```python
from build123d import *

# Parameters (mm, degrees)
BOSS_EXTRUDE1_DEPTH = 6.5
SKETCH4_R           = 1.5875
CUT_EXTRUDE1_DEPTH  = 10
SKETCH5_R           = 1.5875
CUT_EXTRUDE2_DEPTH  = 10


with BuildPart() as part:
    # Sketch3 → Boss-Extrude1 (new body, symmetric)
    with BuildSketch(Plane.XY):
        Polygon((3.175, -3.175), (-4.7625, -3.175), (-4.7625, -4.7625), (4.7625, -4.7625), (4.7625, 4.7625), (3.175, 4.7625), align=None)
    extrude(amount=BOSS_EXTRUDE1_DEPTH, both=True)

    # Sketch4 → Cut-Extrude1 (cut)
    with BuildSketch(Plane(origin=(4.7625, 0, 0), x_dir=(0, 0, -1), z_dir=(1, 0, 0))):
        with Locations((3, 1.2375)):
            Circle(SKETCH4_R)
    extrude(amount=-CUT_EXTRUDE1_DEPTH, mode=Mode.SUBTRACT)

    # Sketch5 → Cut-Extrude2 (cut)
    with BuildSketch(Plane.XZ.offset(4.7625)):
        with Locations((-1.2375, 3)):
            Circle(SKETCH5_R)
    extrude(amount=-CUT_EXTRUDE2_DEPTH, mode=Mode.SUBTRACT)


solid = part.part
```
Work out the finished part from the listing and answer in its coordinate system (mm). A direction names the side the tool comes from. Coordinates: 2 decimals unless noted, no trailing zeros. Write each loop counter-clockwise with the first axis right and the second up, starting at its lowest first coordinate (ties: lowest second). Pieces come first, ordered by that corner, then holes.
Q1. Which of the six approach directions +Z, -Z, +X, -X, +Y, -Y give full straight-line access (tool end or side, diameter ignored) to faces 1 (the face through (3.175, 1, 0)), 2 (the face through (4, 4.762, 0))?
Q2. Each of these flat-tipped pins is pushed along its axis until it touches: pin 1 Ø4 at (x, z) = (-2, -1) entering from +Y (3 decimals); pin 2 Ø3.5 at (x, z) = (-1.24, 3) entering from -Y; pin 3 Ø1 at (y, z) = (-1, 1) entering from -X (3 decimals). Where does it stop, or does it pass through?
Q3. A cutting plane is placed at B-B, the plane y = 0. Give the vertices of the cut face in (x, z) (1 decimal).
Q4. Find the intervals of material crossed by line 1 (X direction, y = -1.5, z = 3.25) (1 decimal); line 2 (Y direction, x = -3, z = 1) (1 decimal), in increasing order.
Q5. A cutting plane is placed at C-C, the plane x = -2.5. Give the vertices of the cut face in (y, z) (1 decimal), then the cut area to 3 significant figures.
Q6. Determine the mould class of faces 3 (the face through (3.98, 1.714, -4.514)), 4 (the face through (4, -2, -6.5)), 5 (the face through (-4.762, -4, 0)), 6 (the face through (-2.823, -3.98, 3.07)) for opening direction Z: released by +Z, released by -Z, zero draft, split by the parting line, or undercut.
Findings below:
1. face 1: +Z, -Z, -X, +Y
1. face 2: +Z, -Z, +X, -X, +Y
2. pin 1: stops at y = -3.175
2. pin 2: stops at y = -4.76
2. pin 3: stops at x = 3.175
3. outline: (3.2, -6.5) - (4.8, -6.5) - (4.8, -4) - (3.2, -4) - close; (3.2, -2) - (4.8, -2) - (4.8, 6.5) - (3.2, 6.5) - close
4. line 1: x = 3.2 to 4.8
4. line 2: y = -4.8 to -3.2
5. outline: (-4.8, -6.5) - (-3.2, -6.5) - (-3.2, 2) - (-4.8, 2) - close; (-4.8, 4) - (-3.2, 4) - (-3.2, 6.5) - (-4.8, 6.5) - close
5. area: 17.6 mm2
6. face 3: undercut
6. face 4: released by -Z
6. face 5: zero draft
6. face 6: undercut
